Input: part model. Units: mm. Frame: model coordinates. A direction names the side the tool comes from. Round coordinates to 2 decimals unless told otherwise and drop trailing zeros. Loops run counter-clockwise (first coordinate to the right, second up) from the corner with the lowest first, then second, coordinate; pieces in that order, holes last.
(1) Cut plane A-A, the plane x = 11.5. Output: boundary loops of the cut face in (y, z).
(2) First-contact query: pin 1 Ø1.8 at (x, y) = (-4.5, 2.5) entering from -Z; pin 2 Ø1.2 at (x, y) = (24.5, 2) entering from +Z; pin 3 Ø1.2 at (x, y) = (-5.5, 2) entering from +Z. Flat tips, straight axial feed; report the tip coordinate or a pass-through.
(3) Draft query along Z for faces 3 (the face through (10, 1, 10)), 4 (the face through (-2.4, 1.9, -1.5)), 5 (the face through (-9.64, 2.86, 0.21)). Return one class per face: released by +Z, released by -Z, zero draft, split by the parting line, or undercut.
(4) Access query for faces 1 (the face through (-10, 1, 0)), 2 (the face through (-7.6, 1.9, -1.5)). Directions: +Z, -Z, +X, -X, +Y, -Y. A direction counts if a zero-diameter tool reaches every point of the face in a straight line with its end or side. Return the directions, or none.
(5) Line query: line 1 (X direction, y = 1.85, z = 0); line 2 (X direction, y = 0.8, z = -1.5); line 3 (Z direction, x = 25, y = 0.4). Output: solid intervals per line, ascending.
(6) Cut plane B-B, the plane y = 1.2. Output: boundary loops of the cut face in (x, z).
from build123d import *

# Parameters (mm, degrees)
BOSS_EXTRUDE1_DEPTH             = 3
M3X0_5_TAPPED_HOLE1_D           = 3
M3X0_5_TAPPED_HOLE1_CSINK_D     = 3.05
M3X0_5_TAPPED_HOLE1_CSINK_ANGLE = 90
CHAMFER1_SIZE                   = 0.5
SKETCH3_R                       = 3
CUT_EXTRUDE1_DEPTH              = 32.764760349
CUT_EXTRUDE2_DEPTH              = 2.3


with BuildPart() as part:
    # Sketch2 → Boss-Extrude1 (new body)
    with BuildSketch(Plane(origin=(0, 0, 0), x_dir=(1, 0, 0), z_dir=(0, 1, 0))):
        with BuildLine():
            Line((0, 10), (20, 10))
            ThreePointArc((20, 10), (30, 0), (20, -10))
            Line((20, -10), (0, -10))
            ThreePointArc((0, -10), (-10, 0), (0, 10))
        make_face()
    extrude(amount=BOSS_EXTRUDE1_DEPTH)

    # M3x0.5 Tapped Hole1 (through all)
    with Locations(Plane(origin=(0, 3, 0), x_dir=(1, 0, 0), z_dir=(0, 1, 0))):
        with Locations((-5, 0), (25, 0)):
            CounterSinkHole(M3X0_5_TAPPED_HOLE1_D / 2, M3X0_5_TAPPED_HOLE1_CSINK_D / 2, counter_sink_angle=M3X0_5_TAPPED_HOLE1_CSINK_ANGLE)

    # Chamfer1
    chamfer1_edges = [part.edges().sort_by_distance(p)[0] for p in [
        (30, 3, 0),
        (10, 3, -10),
        (-10, 3, 0),
        (10, 0, -10),
        (30, 0, 0),
        (10, 0, 10),
        (-10, 0, 0),
        (10, 3, 10),
    ]]
    chamfer(chamfer1_edges, length=CHAMFER1_SIZE)

    # Sketch3 → Cut-Extrude1 (cut, through all)
    with BuildSketch(Plane(origin=(0, 3, 0), x_dir=(1, 0, 0), z_dir=(0, 1, 0))):
        with Locations(Location((10, 0, 0), (0, 0, 270))):
            Circle(SKETCH3_R)
    extrude(amount=-CUT_EXTRUDE1_DEPTH, mode=Mode.SUBTRACT)

    # Sketch16 → Cut-Extrude2 (cut)
    with BuildSketch(Plane(origin=(0, 3, 0), x_dir=(1, 0, 0), z_dir=(0, 1, 0))):
        Polygon((-1.535898385, 0), (-3.267949192, 3), (-6.732050808, 3), (-8.464101615, 0), (-6.732050808, -3), (-3.267949192, -3), align=None)
        Polygon((21.535898385, 0), (23.267949192, -3), (26.732050808, -3), (28.464101615, 0), (26.732050808, 3), (23.267949192, 3), align=None)
    extrude(amount=-CUT_EXTRUDE2_DEPTH, mode=Mode.SUBTRACT)


solid = part.part
Reported:
1. outline: (0, -9.5) - (0.5, -10) - (2.5, -10) - (3, -9.5) - (3, -2.6) - (0, -2.6) - close; (0, 2.6) - (3, 2.6) - (3, 9.5) - (2.5, 10) - (0.5, 10) - (0, 9.5) - close
2. pin 1: stops at z = -9.33
2. pin 2: stops at z = 9.21
2. pin 3: stops at z = 8.72
3. face 3: released by +Z
3. face 4: undercut
3. face 5: split by the parting line
4. face 1: -X, +Y, -Y
4. face 2: +Y
5. line 1: x = -10 to -8.46, -1.54 to 7, 13 to 21.54, 28.46 to 30
5. line 2: x = -9.89 to -7.6, -2.4 to 7.4, 12.6 to 22.4, 27.6 to 29.89
5. line 3: z = -8.54 to -1.5, 1.5 to 8.54
6. outline: (0, -10) - (20, -10) arc R10 ccw to (20, 10) - (0, 10) arc R10 ccw to start; hole (-8.46, 0) - (-6.73, -3) - (-3.27, -3) - (-1.54, 0) - (-3.27, 3) - (-6.73, 3) - close; hole circle Ø6 at (10, 0); hole (21.54, 0) - (23.27, -3) - (26.73, -3) - (28.46, 0) - (26.73, 3) - (23.27, 3) - close
